Geometry: final body of the model. Coordinates: model frame, mm. Coordinates: 2 decimals unless noted, no trailing zeros. Order: outer loops, then holes, each group sorted by start corner. A loop starts at its lowest first (then second) coordinate and runs counter-clockwise, first axis right, second up. Notation, with made-up numbers: (21.25, -28.75) - (50.25, -28.75) arc R17 ccw to (50.25, -12.75) - close; hole circle Ø4 at (32.5, -8). An arc over 180 degrees is marked (long way). Use a Markdown table: item, result. Add a question column.
Autodesk Inventor part; units mm, degrees
ref_plane "YZ Plane" through (0, 0, 0) normal (1, 0, 0) x (0, 1, 0)
ref_plane "XZ Plane" through (0, 0, 0) normal (0, 1, 0) x (-1, 0, 0)
ref_plane "XY Plane" through (0, 0, 0) normal (0, 0, 1) x (1, 0, 0)
sketch "Sketch3" plane through (0, 0, 0) normal (0, 1, 0) x (-1, 0, 0)
  circle A0 centre (11.1125, 0) radius 1.4906
  circle A1 centre (-5.5563, 9.6237) radius 1.4906
  circle A2 centre (-5.5562, -9.6237) radius 1.4906
  circle A3 centre (0, 0) radius 5.25
  line L0 (0, 0) -> (11.1125, 0)
  line L1 (0, 0) -> (-5.5563, 9.6237)
  line L2 (0, 0) -> (-5.5562, -9.6237)
  line L3 (0, 11.7306) -> (0, -34.9786)
  line L4 (38.6398, 0) -> (-3.2951, 0)
  circle A4 centre (40, 0) radius 5.05
  circle A5 centre (0, -40) radius 5.05
  circle A6 centre (0, 40) radius 5.05
  circle A7 centre (-40, 0) radius 5.05
  line L5 (-47.625, -47.625) -> (47.625, -47.625)
  line L6 (47.625, -47.625) -> (47.625, 47.625)
  line L7 (47.625, 47.625) -> (-47.625, 47.625)
  line L8 (-47.625, 47.625) -> (-47.625, -47.625)
  line L9 (-47.625, -47.625) -> (47.625, 47.625) construction
  line L10 (47.625, -47.625) -> (-47.625, 47.625) construction
  dimension "d19" = 120
  dimension "d20" = 120
  dimension "d21" = 11.1125
  dimension "d22" = 11.1125
  dimension "d23" = 11.1125
  dimension "d24" = 2.9811
  dimension "d25" = 2.9811
  dimension "d26" = 2.9811
  dimension "d27" = 80
  dimension "d28" = 80
  dimension "d29" = 10.1
  dimension "d30" = 10.1
  dimension "d31" = 95.25
  dimension "d32" = 95.25
  dimension "d36" = 10.5
extrude "Extrusion6" add sketch "Sketch3" along normal blind 6.35
fillet "Fillet1" radius 25.4 4 edges at (-47.625, 3.175, 47.625) (47.625, 3.175, 47.625) (47.625, 3.175, -47.625) (-47.625, 3.175, -47.625)
equation "\"d22\" = d21"
equation "\"d23\" = d21"
equation "\"d25\" = d24"
equation "\"d26\" = d24"
equation "\"d28\" = d27"
equation "\"d30\" = d29"
equation "\"d32\" = d31"
properties part number "Vertical_Lead_Screw_Plate"
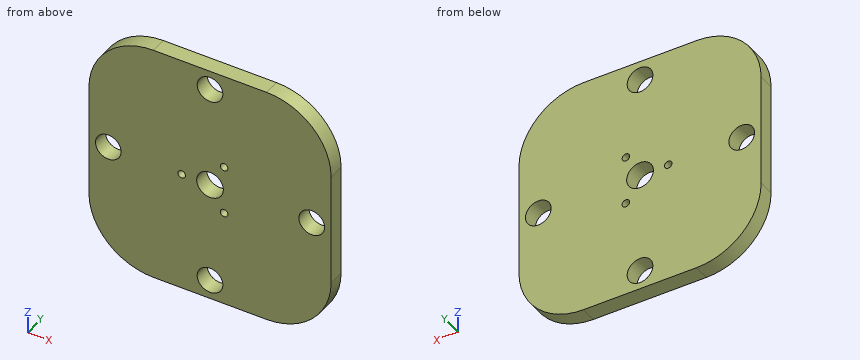
1) Section B-B (x = 40). Return loops of the section in (y, z).
2) Section C-C (z = 40). Return loops of the section in (x, y), then the cut area to 3 significant figures.
3) Ray query, line 1 along Z through (x, y) = (-0.5, 4.75) (3 decimals); line 2 along X through (y, z) = (5.75, -39); line 3 along X through (y, z) = (2, -1) (3 decimals). Return the intervals inside material, ascending.
4) Pin query (flat end, axial travel): pin 1 (13 mm diameter, centred on x = -40, z = 0, fed in from +Y); pin 2 (2 mm diameter, centred on y = 2, z = 38, fed in from +X). Return the tip coordinate at first contact, or that it passes through.
5) Section A-A (z = 0). Return loops of the section in (x, y) (3 decimals).
6) Section D-D (y = 4.5). Give the number of separate pieces and of enclosed holes in the cut face, then the cut area to 3 significant figures.
Values follow:
| question | item | result |
|---|---|---|
| 1 | outline | (0, -40.37) - (6.35, -40.37) - (6.35, -5.05) - (0, -5.05) - close; (0, 5.05) - (6.35, 5.05) - (6.35, 40.37) - (0, 40.37) - close |
| 2 | outline | (-40.37, 0) - (-5.05, 0) - (-5.05, 6.35) - (-40.37, 6.35) - close; (5.05, 0) - (40.37, 0) - (40.37, 6.35) - (5.05, 6.35) - close |
| 2 | area | 449 mm² |
| 3 | line 1 | z = -47.625 to -45.025, -34.975 to -5.226, 5.226 to 34.975, 45.025 to 47.625 |
| 3 | line 2 | x = -41.3 to -4.95, 4.95 to 41.3 |
| 3 | line 3 | x = -47.625 to -44.95, -35.05 to -12.218, -10.007 to -5.154, 5.154 to 35.05, 44.95 to 47.625 |
| 4 | pin 1 | stops at y = 6.35 |
| 4 | pin 2 | stops at x = 42.89 |
| 5 | outline | (-47.625, 0) - (-45.05, 0) - (-45.05, 6.35) - (-47.625, 6.35) - close; (-34.95, 0) - (-12.603, 0) - (-12.603, 6.35) - (-34.95, 6.35) - close; (-9.622, 0) - (-5.25, 0) - (-5.25, 6.35) - (-9.622, 6.35) - close; (5.25, 0) - (34.95, 0) - (34.95, 6.35) - (5.25, 6.35) - close; (45.05, 0) - (47.625, 0) - (47.625, 6.35) - (45.05, 6.35) - close |
| 6 | separate pieces | 1 |
| 6 | enclosed holes | 8 |
| 6 | area | 8,090 mm² |
